```python
from build123d import *

# Parameters (mm, degrees)
SKIZZE1_W                       = 140
SKIZZE1_H                       = 20
AUFSATZ_LINEAR_AUSTRAGEN1_DEPTH = 6
SKIZZE2_W                       = 10
SKIZZE2_H                       = 4
AUFSATZ_LINEAR_AUSTRAGEN2_DEPTH = 6
SCHNITT_LINEAR_AUSTRAGEN1_REACH = 8
SKIZZE3_W                       = 3.8
SKIZZE3_H                       = 10
SCHNITT_LINEAR_AUSTRAGEN2_REACH = 8


with BuildPart() as part:
    # Skizze1 → Aufsatz-Linear austragen1 (new body)
    with BuildSketch(Plane.XY):
        with Locations((70, 10)):
            Rectangle(SKIZZE1_W, SKIZZE1_H)
    extrude(amount=AUFSATZ_LINEAR_AUSTRAGEN1_DEPTH)

    # Skizze2 → Aufsatz-Linear austragen2 (add)
    with BuildSketch(Plane(origin=(0, 0, 0), x_dir=(-1, 0, 0), z_dir=(0, 0, -1))):
        with Locations((-135, 22)):
            Rectangle(SKIZZE2_W, SKIZZE2_H)
        with Locations((-115, 22)):
            Rectangle(SKIZZE2_W, SKIZZE2_H)
    extrude(amount=-AUFSATZ_LINEAR_AUSTRAGEN2_DEPTH)

    # Skizze3 → Schnitt-Linear austragen1 (cut, up to next)
    with BuildSketch(Plane(origin=(0, 0, 0), x_dir=(-1, 0, 0), z_dir=(0, 0, -1)), mode=Mode.PRIVATE) as schnitt_linear_austragen1_sk1:
        with Locations((-4.9, 15)):
            Rectangle(SKIZZE3_W, SKIZZE3_H)
    schnitt_linear_austragen1_tool1 = extrude(schnitt_linear_austragen1_sk1.sketch, amount=-SCHNITT_LINEAR_AUSTRAGEN1_REACH, mode=Mode.PRIVATE) & part.part
    add(schnitt_linear_austragen1_tool1.solids().sort_by_distance((4.9, 15, 0))[0], mode=Mode.SUBTRACT)

    # Skizze4 → Schnitt-Linear austragen2 (cut, up to next)
    with BuildSketch(Plane.XY.offset(6), mode=Mode.PRIVATE) as schnitt_linear_austragen2_sk1:
        with BuildLine():
            Line((134.01576743, 8.6), (65, 8.6))
            ThreePointArc((65, 8.6), (61.747308807, 7.252691193), (60.4, 4))
            ThreePointArc((60.4, 4), (59.228427125, 1.171572875), (56.4, 0))
            Line((56.4, 0), (140, 0))
            Line((140, 0), (140, 14.58423257))
            ThreePointArc((140, 14.58423257), (138.247258861, 10.352741139), (134.01576743, 8.6))
        make_face()
    schnitt_linear_austragen2_tool1 = extrude(schnitt_linear_austragen2_sk1.sketch, amount=-SCHNITT_LINEAR_AUSTRAGEN2_REACH, mode=Mode.PRIVATE) & part.part
    add(schnitt_linear_austragen2_tool1.solids().sort_by_distance((100.680271, 4.324252, 6))[0], mode=Mode.SUBTRACT)


solid = part.part
```
Could you check a few things on this model? Use its own coordinates, in mm. A direction names the side the tool comes from. Give positions to 0.01 mm unless a question says otherwise; leave off trailing zeros. Loops run counter-clockwise (first coordinate to the right, second up) from the corner with the lowest first, then second, coordinate; pieces in that order, holes last. Notation, with made-up numbers: (-28, 14) -> (-7, 14) arc R23 ccw to (-7, 42) -> close; hole circle Ø3 at (61, -39.5). An arc over 180 degrees is marked (long way). Put each result on its own line as item: value.
(1) Please list where these lines run through material, in increasing order: probe 1 along X at (y, z) = (19.25, 2.9); probe 2 along X at (y, z) = (22.5, 0.8); probe 3 along Y at (x, z) = (19, 4.95). Write a range as [from, to].
Computed:
probe 1: [0, 3], [6.8, 140]
probe 2: [110, 120], [130, 140]
probe 3: [0, 20]
(2) For faces 1 (the face through (1, 20, 3)), 2 (the face through (100, 8.6, 3)), 3 (the face through (125, 20, 3)), 4 (the face through (140, 19, 3)), 5 (the face through (28, 0, 3)), which set-ups out of +Z, -Z, +X, -X, +Y, -Y let a thin tool reach every point of the face, with its end or its side?
Computed:
face 1: +Z, -Z, -X, +Y
face 2: +Z, -Z, +X, -Y
face 3: +Z, -Z, +Y
face 4: +Z, -Z, +X, +Y, -Y
face 5: +Z, -Z, +X, -X, -Y
(3) Thinking about a two-plate mould opening in X: for faces 6 (the face through (138.294, 10.4, 3.042)), 7 (the face through (3, 15, 3)), 8 (the face through (110, 22, 3)), which applies, pulls with the +X half, pulls with the -X half, needs draft (parallel to the pull), parting line crosses it, or undercut?
Computed:
face 6: pulls with the +X half
face 7: undercut
face 8: pulls with the -X half
(4) Imagine slicing it at C-C on x = 38.5. Write out the boundary of the cut face in (y, z), plus the area to 3 significant figures.
Computed:
outline: (0, 0) -> (20, 0) -> (20, 6) -> (0, 6) -> close
area: 120 mm^2
(5) Imagine slicing it at D-D on y = 6.25. Write out the boundary of the cut face in (x, z).
Computed:
outline: (0, 0) -> (60.99, 0) -> (60.99, 6) -> (0, 6) -> close
(6) I'm going to push flat-ended pins straight in: pin 1 Ø3 at (x, z) = (41, 2.5) entering from +Y; pin 2 Ø1.2 at (y, z) = (21.5, 2) entering from -X; pin 3 Ø3 at (x, z) = (91.5, 1.5) entering from -Y. Where does each tip first touch, or does it pass through?
Computed:
pin 1: y = 20
pin 2: x = 110
pin 3: y = 8.6
(7) Imagine slicing it at B-B on z = 2.4. Write out the boundary of the cut face in (x, y), plus the area to 3 significant figures.
Computed:
outline: (0, 0) -> (56.4, 0) arc R4 ccw to (60.4, 4) arc R4.6 cw to (65, 8.6) -> (134.02, 8.6) arc R5.98 ccw to (140, 14.58) -> (140, 24) -> (130, 24) -> (130, 20) -> (120, 20) -> (120, 24) -> (110, 24) -> (110, 20) -> (6.8, 20) -> (6.8, 10) -> (3, 10) -> (3, 20) -> (0, 20) -> close
area: 2,150 mm^2
(8) Imagine slicing it at A-A on y = 22.25. Write out the boundary of the cut face in (x, z).
Computed:
outline: (110, 0) -> (120, 0) -> (120, 6) -> (110, 6) -> close; (130, 0) -> (140, 0) -> (140, 6) -> (130, 6) -> close
